Geometry check sheet. Reference: drawing and pictorial views, mm from the part's lowest x, y, z. Round coordinates to 2 decimals unless told otherwise and drop trailing zeros. Order: outer loops, then holes, each group sorted by start corner. A loop starts at its lowest first (then second) coordinate and runs counter-clockwise, first axis right, second up. Notation, with made-up numbers: M 34.5,3 L 82.5,3 A28 cw 82.5,38 Z; hole C -10,12 d3. An arc over 180 degrees is marked long. Answer as a JSON object with one key per item and string values. Group by question number.
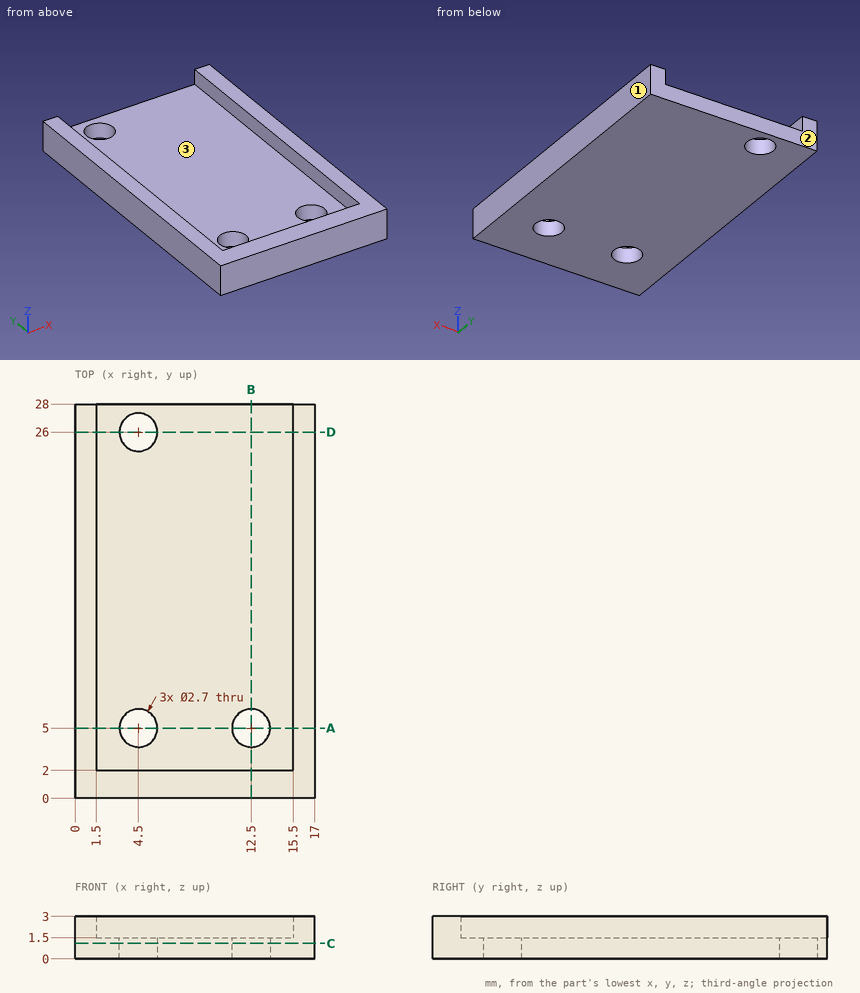
Q1. Gauge pin test, flat ends, axial feed: pin 1 Ø10 at (x, y) = (15, 18) entering from -Z; pin 2 Ø2.5 at (x, y) = (4.5, 26) entering from +Z; pin 3 Ø5 at (x, y) = (4.5, 6) entering from +Z. Record the tip position at first contact, or that the pin passes through.
Q2. Cross-section at D-D, the plane y = 26. Record the cut outline in (x, z).
Q3. Cross-section at A-A, the plane y = 5. Record the cut outline in (x, z).
Q4. Thickness scan on line 1 (Y direction, x = 4.5, z = 0.75); line 2 (X direction, y = 24, z = 1.65); line 3 (Y direction, x = 12.5, z = 0.6). Record the ranges inside material, lowest first. Write a range as from..to.
Q5. Cross-section at B-B, the plane x = 12.5. Record the cut outline in (y, z), then the cut area to 4 significant figures.
Q6. Release check for a two-part mould opening along X. For the marked faces 1, 2 and 3 record: released by +X, released by -X, zero draft, split by the parting line, or undercut.
Q7. Cross-section at C-C, the plane z = 1.1. Record the cut outline in (x, y), then the cut area to 3 significant figures.
Conclusion:
{
 "1": {"pin 1": "z = 0", "pin 2": "through", "pin 3": "z = 1.5"},
 "2": {"outline": "M 0,0 L 3.15,0 L 3.15,1.5 L 1.5,1.5 L 1.5,3 L 0,3 Z; M 5.85,0 L 17,0 L 17,3 L 15.5,3 L 15.5,1.5 L 5.85,1.5 Z"},
 "3": {"outline": "M 0,0 L 3.15,0 L 3.15,1.5 L 1.5,1.5 L 1.5,3 L 0,3 Z; M 5.85,0 L 11.15,0 L 11.15,1.5 L 5.85,1.5 Z; M 13.85,0 L 17,0 L 17,3 L 15.5,3 L 15.5,1.5 L 13.85,1.5 Z"},
 "4": {"line 1": "0..3.65, 6.35..24.65, 27.35..28", "line 2": "0..1.5, 15.5..17", "line 3": "0..3.65, 6.35..28"},
 "5": {"outline": "M 0,0 L 3.65,0 L 3.65,1.5 L 2,1.5 L 2,3 L 0,3 Z; M 6.35,0 L 28,0 L 28,1.5 L 6.35,1.5 Z", "area": "40.95 mm2"},
 "6": {"face 1": "released by +X", "face 2": "zero draft", "face 3": "undercut"},
 "7": {"outline": "M 0,0 L 17,0 L 17,28 L 0,28 Z; hole C 4.5,5 d2.7; hole C 4.5,26 d2.7; hole C 12.5,5 d2.7", "area": "459 mm2"}
}
